Work out the finished part from the listing and answer in its coordinate system (mm). Coordinates: 2 decimals unless noted, no trailing zeros. Write each loop counter-clockwise with the first axis right and the second up, starting at its lowest first coordinate (ties: lowest second). Pieces come first, ordered by that corner, then holes. Notation, with made-up numbers: (44, 31) - (80, 31) arc R28 cw to (80, 51) - close; hole circle Ø10 at (-10, -5.5). An arc over 180 degrees is marked (long way). Use one line per item in the form item = value. Start each with the question number.
Item 1: A cutting plane is placed at B-B (z = 0.65). Write down the section's boundary in (x, y).
Item 2: A cutting plane is placed at C-C (y = 5.25). Write down the section's boundary in (x, z), then the cut area to 3 significant figures.
Item 3: Given pin 1 (5.5 mm diameter, centred on x = -4.29, y = 6.5, fed in from +Z); pin 2 (3 mm diameter, centred on x = -11.5, y = 8.5, fed in from -Z), each flat-ended and moving along its own axis, determine where each tip first touches the part or whether it passes through.
Item 4: A cutting plane is placed at A-A (x = -6). Write down the section's boundary in (y, z).
Item 5: A cutting plane is placed at D-D (y = 17). Write down the section's boundary in (x, z), then the cut area to 3 significant figures.
Item 6: Consider probe 1 along Y at (x, z) = (-19, 0.25); probe 2 along Y at (x, z) = (-3.5, 1.3); probe 3 along Z at (x, y) = (-6.25, 15.75). Determine where each line is inside the solid, lowest interval first.
Item 7: Determine the mould class of faces 1 (the cylindrical face through (-21.614, 18.84, 0.805)), 2 (the flat face through (-20, 16, 1.588)), 3 (the cylindrical face through (-6.07, 7.636, 0.803)), 4 (the flat face through (0, 4, 1)) for opening direction X: released by +X, released by -X, zero draft, split by the parting line, or undercut.
Autodesk Inventor part; units mm, degrees
ref_plane "YZ Plane" through (0, 0, 0) normal (1, 0, 0) x (0, 1, 0)
ref_plane "XZ Plane" through (0, 0, 0) normal (0, 1, 0) x (-1, 0, 0)
ref_plane "XY Plane" through (0, 0, 0) normal (0, 0, 1) x (1, 0, 0)
sketch "Sketch1" plane through (0, 0, 0) normal (0, 0, 1) x (1, 0, 0)
  line L0 (0, 0) -> (-4.699, 0)
  line L1 (-4.699, 0) -> (-14.3764, 13.4874)
  line L2 (-14.3764, 13.4874) -> (-21.9964, 13.4874)
  line L3 (-21.9964, 13.4874) -> (-21.9964, 19.2024)
  line L4 (-21.9964, 19.2024) -> (-8.3105, 19.2024)
  line L5 (-8.3105, 19.2024) -> (0, 7.62)
  line L6 (0, 7.62) -> (0, 0)
  line L7 (0, 23.0429) -> (0, -3.8405)
  line L8 (-26.3957, 0) -> (4.3993, 0)
  dimension "d0" = 7.62
  dimension "d1" = 5.715
  dimension "d2" = 4.699
  dimension "d3" = 19.2024
  dimension "d4" = 21.9964
  dimension "d5" = 7.62
  dimension "d6" = 13.6859
  dimension "d7" = 14.2554
extrude "Extrusion1" add sketch "Sketch1" along normal blind 1.5875
sketch "Sketch2" plane through (0, 0, 0) normal (0, 0, 1) x (1, 0, 0)
  circle A0 centre (-4.2926, 6.5024) radius 0.635
  line L0 (-26.3957, 0) -> (4.3993, 0)
  line L1 (0, 23.0429) -> (0, -3.8405)
  line L2 (-21.9964, 13.4874) -> (-21.9964, 19.2024)
  line L3 (-21.9964, 19.2024) -> (-8.3105, 19.2024)
  point P0 (0, 0)
  dimension "d11" = 17.7038
  dimension "d12" = 12.7
  dimension "d13" = 1.27
hole "Hole1" at (-4.2926, 6.5024, 0) direction (0, 0, 1) diameter 4.2164 end through all
fillet "Fillet1" radius 1.27 6 edges at (-21.9964, 13.4874, 0.7937) (-14.3764, 13.4874, 0.7937) (-4.699, 0, 0.7937) (0, 7.62, 0.7937) (-8.3105, 19.2024, 0.7937) (-21.9964, 19.2024, 0.7937)
fillet "Fillet2" radius 0.254 1 edges at (0, 0, 0.7937)
sketch "Sketch3" plane through (0, 0, 1.5875) normal (0, 0, 1) x (1, 0, 0)
  line L0 (-20.7264, 19.2024) -> (-8.9624, 19.2024)
  circle A0 centre (-4.2926, 6.5024) radius 2.1082
  line L1 (0, 0) -> (-18.8214, 0)
  line L2 (-18.8214, 0) -> (-18.8214, 19.2024)
  line L3 (-18.8214, 19.2024) -> (0, 19.2024)
  line L4 (0, 19.2024) -> (0, 0)
  point P0 (-21.9964, 17.9324)
  dimension "d23" = 3.175
extrude "Extrusion2" cut sketch "Sketch3" against normal blind 0.127
sketch "Sketch4" plane through (0, 0, 0) normal (0, 0, -1) x (-1, 0, 0)
  circle A0 centre (4.2926, 6.5024) radius 2.1082
  line L0 (21.9964, 14.7574) -> (21.9964, 17.9324)
  line L1 (20.7264, 19.2024) -> (8.9624, 19.2024)
  line L2 (0, 0) -> (18.8214, 0)
  line L3 (18.8214, 0) -> (18.8214, 19.2024)
  line L4 (18.8214, 19.2024) -> (0, 19.2024)
  line L5 (0, 19.2024) -> (0, 0)
  dimension "d26" = 3.175
extrude "Extrusion3" cut sketch "Sketch4" against normal blind 0.127
fillet "Fillet3" radius 1.27 4 edges at (-18.8214, 13.4874, 0.0635) (-18.8214, 19.2024, 0.0635) (-18.8214, 19.2024, 1.524) (-18.8214, 13.4874, 1.524)
properties part number "J002856" material "STAINLESS STEEL, 303"
Answer:
q1.outline = (-22, 14.76) arc R1.27 ccw to (-20.73, 13.49) - (-15.03, 13.49) arc R1.27 cw to (-14, 12.96) - (-5.08, 0.53) arc R1.27 ccw to (-4.05, 0) - (-0.25, 0) arc R0.25 ccw to (0, 0.25) - (0, 7.21) arc R1.27 ccw to (-0.24, 7.95) - (-7.93, 18.67) arc R1.27 ccw to (-8.96, 19.2) - (-20.73, 19.2) arc R1.27 ccw to (-22, 17.93) - close; hole circle Ø4.22 at (-4.29, 6.5)
q2.outline = (-8.47, 0.13) - (-5.99, 0.13) - (-5.99, 1.46) - (-8.47, 1.46) - close; (-2.6, 0.13) - (0, 0.13) - (0, 1.46) - (-2.6, 1.46) - close
q2.area = 6.77 mm²
q3.pin_1 = 1.46
q3.pin_2 = 0.13
q4.outline = (1.81, 0.13) - (5.27, 0.13) - (5.27, 1.46) - (1.81, 1.46) - close; (7.74, 0.13) - (15.98, 0.13) - (15.98, 1.46) - (7.74, 1.46) - close
q5.outline = (-22, 0) - (-18.82, 0) - (-18.82, 0.13) - (-6.73, 0.13) - (-6.73, 1.46) - (-18.82, 1.46) - (-18.82, 1.59) - (-22, 1.59) - close
q5.area = 21.2 mm²
q6.probe_1 = 13.49 to 19.2
q6.probe_2 = 0 to 4.55, 8.46 to 12.5
q6.probe_3 = 0.13 to 1.46
q7.face_1 = released by -X
q7.face_2 = zero draft
q7.face_3 = undercut
q7.face_4 = released by +X
